Input: part model. Units: mm. Frame: model coordinates. Face numbers are marked on the shaded views. A direction names the side the tool comes from. Coordinates: 2 decimals unless noted, no trailing zeros. Order: outer loops, then holes, each group sorted by start corner. A loop starts at its lowest first (then second) coordinate and runs counter-clockwise, first axis right, second up. Notation, with made-up numbers: M 80.5,14.25 L 96.5,14.25 A14 cw 96.5,18.25 Z; hole C 18,-31.75 d11. An arc over 180 degrees is marked long. Answer in a Markdown table with one row per item.
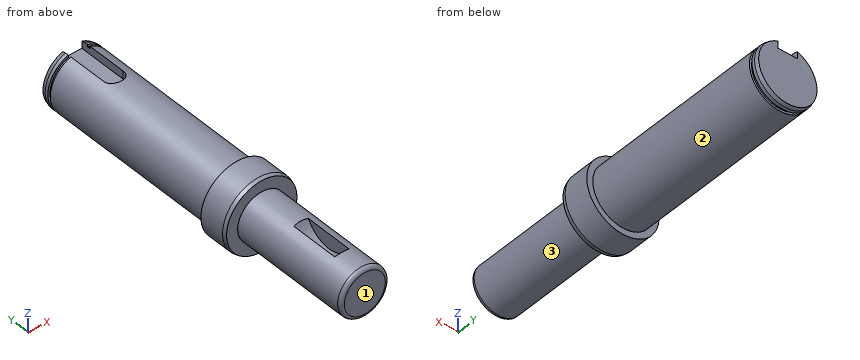
from build123d import *

# Parameters (mm, degrees)
F0_R      = 12.5
F1_DEPTH  = 80
F2_R      = 15
F3_DEPTH  = 12
F4_R      = 10
F5_DEPTH  = 50
F6_SIZE2  = 1.492820323
F6_SIZE   = 0.4
F7_SIZE2  = 1.492820323
F7_SIZE   = 0.4
F8_R      = 1.5
F11_DEPTH = 4
F12_W     = 1.2
F12_H     = 0.9
F14_R     = 11
F15_DEPTH = 3


with BuildPart() as f1:
    # F0 (on Front) → F1 (new body)
    with BuildSketch(Plane.XZ):
        Circle(F0_R)
    extrude(amount=F1_DEPTH)

    # F2 (on face) → F3 (join)
    with BuildSketch(Plane.XZ.offset(80)):
        Circle(F2_R)
    extrude(amount=F3_DEPTH)

    # F4 (on face) → F5 (join)
    with BuildSketch(Plane.XZ.offset(92)):
        Circle(F4_R)
    extrude(amount=F5_DEPTH)

    # F6
    f6_edges = [f1.edges().sort_by_distance(p)[0] for p in [
        (-12.5, 0, 0),
    ]]
    f6_side = f1.faces().sort_by_distance((0, 0, 0))[0]
    chamfer(f6_edges, length=F6_SIZE, length2=F6_SIZE2, reference=f6_side)

    # F7
    f7_edges = [f1.edges().sort_by_distance(p)[0] for p in [
        (-15, -92, 0),
    ]]
    f7_side = f1.faces().sort_by_distance((-14.575736, -92, 0))[0]
    chamfer(f7_edges, length=F7_SIZE, length2=F7_SIZE2, reference=f7_side)

    # F8
    f8_edges = [f1.edges().sort_by_distance(p)[0] for p in [
        (-10, -142, 0),
    ]]
    fillet(f8_edges, radius=F8_R)

    # F10 (on offset) → F11 (cut)
    with BuildSketch(Plane.XY.offset(12.5)):
        with BuildLine():
            Line((-4, 31.7779608309), (-4, -20))
            ThreePointArc((-4, -20), (0, -24), (4, -20))
            Line((4, -20), (4, 31.7779608309))
            Line((4, 31.7779608309), (-4, 31.7779608309))
        make_face()
    extrude(amount=-F11_DEPTH, mode=Mode.SUBTRACT)

    # F12 (on Right) → F13 (revolve, cut)
    with BuildSketch(Plane.YZ):
        with Locations((-3.4, -12.05)):
            Rectangle(F12_W, F12_H)
    revolve(axis=Axis((0, 0, 0), (0, 1, 0)), mode=Mode.SUBTRACT)

    # F14 (on Right) → F15 (cut, symmetric)
    with BuildSketch(Plane.YZ):
        with Locations((-121, 14.4)):
            Circle(F14_R)
    extrude(amount=F15_DEPTH, both=True, mode=Mode.SUBTRACT)


solid = f1.part
1) Contact query for flat-ended pins moving along their axis: pin 1 (3.5 mm diameter, centred on y = -5, z = 10.5, fed in from -X); pin 2 (2 mm diameter, centred on x = 5, y = -104, fed in from +Z); pin 3 (8 mm diameter, centred on y = -63, z = -1, fed in from +X). Output: stop coordinate, or through.
Resolved:
| item | result |
|---|---|
| pin 1 | stops at x = -8.93 |
| pin 2 | stops at z = 9.17 |
| pin 3 | stops at x = 12.5 |
2) Cut plane A-A, the plane z = 0. Output: boundary loops of the cut face in (x, y), and give its area (3 significant figures).
Resolved:
| item | result |
|---|---|
| outline | M -15,-90.51 L -14.6,-92 L -10,-92 L -10,-140.5 A1.5 ccw -8.5,-142 L 8.5,-142 A1.5 ccw 10,-140.5 L 10,-92 L 14.6,-92 L 15,-90.51 L 15,-80 L 12.5,-80 L 12.5,-4 L 11.6,-4 L 11.6,-2.8 L 12.5,-2.8 L 12.5,-1.49 L 12.1,0 L -12.1,0 L -12.5,-1.49 L -12.5,-2.8 L -11.6,-2.8 L -11.6,-4 L -12.5,-4 L -12.5,-80 L -15,-80 Z |
| area | 3,360 mm2 |
3) Cut plane B-B, the plane x = 0. Output: boundary loops of the cut face in (y, z), and give its area (3 significant figures).
Resolved:
| item | result |
|---|---|
| outline | M -142,-8.5 A1.5 ccw -140.5,-10 L -92,-10 L -92,-14.6 L -90.51,-15 L -80,-15 L -80,-12.5 L -4,-12.5 L -4,-11.6 L -2.8,-11.6 L -2.8,-12.5 L -1.49,-12.5 L 0,-12.1 L 0,8.5 L -24,8.5 L -24,12.5 L -80,12.5 L -80,15 L -90.51,15 L -92,14.6 L -92,10 L -110.92,10 A11 cw -131.08,10 L -140.5,10 A1.5 ccw -142,8.5 Z |
| area | 3,170 mm2 |
4) Material intervals for probe 1 along Y at (x, z) = (-10.5, 5.25); probe 2 along Y at (x, z) = (12.25, -3.25); probe 3 along X at (y, z) = (-118.5, 0.5), sorted ascending.
Resolved:
| item | result |
|---|---|
| probe 1 | y = -92 to -4, -2.8 to 0 |
| probe 2 | y = -92 to -80 |
| probe 3 | x = -9.99 to 9.99 |
5) Cut plane C-C, the plane y = -43.5. Output: boundary loops of the cut face in (x, z).
Resolved:
| item | result |
|---|---|
| outline | C 0,0 d25 |
6) Reachability of the marked faces 1, 2 and 3 from +Z, -Z, +X, -X, +Y, -Y: full face, straight path, thin tool, end or side. Return the list, or none.
Resolved:
| item | result |
|---|---|
| face 1 | +Z, -Z, +X, -X, -Y |
| face 2 | +Y |
| face 3 | -Y |
7) Cut plane D-D, the plane y = -15. Output: boundary loops of the cut face in (x, z).
Resolved:
| item | result |
|---|---|
| outline | M -4,8.5 L -4,11.84 A12.5 ccw long 4,11.84 L 4,8.5 Z |
